The drawing under review shows one solid part. Ordinate dimensions are in mm from its lowest x, y, z. A direction names the side the tool comes from. Give positions to 0.01 mm unless a question says otherwise; leave off trailing zeros. Loops run counter-clockwise (first coordinate to the right, second up) from the corner with the lowest first, then second, coordinate; pieces in that order, holes last. Notation, with made-up numbers: M -6.75,33 L 44.25,33 A6 cw 44.25,41 Z; hole C -9.5,-2.5 d4. An arc over 180 degrees is marked long. Write item = value, one per line. Start each with the question number.
1. For the marked faces 4, 5 and 6, list the 3-axis set-ups (+Z, -Z, +X, -X, +Y, -Y) from which the entire face can be reached by the end or side of a thin tool; tool diameter is ignored.
2. We need section D-D on x = 9.5. Give the boundary of the cut face in (y, z).
3. We need section A-A on z = 8.5. Give the boundary of the cut face in (x, y), then the cut area to 3 significant figures.
4. For pin 1 (1.5 mm diameter, centred on x = 12, y = 42.5, fed in from -Z); pin 2 (12 mm diameter, centred on x = 11.5, y = 18.5, fed in from -Z); pin 3 (1 mm diameter, centred on x = 15, y = 39.5, fed in from +Z), all flat-tipped, find the tip position at first contact; note any pin that passes through.
5. Wall thickness on line 1 along X through (y, z) = (3.5, 8.5); line 2 along Z through (x, y) = (1.5, 19.5); line 3 along Z through (x, y) = (10.25, 11): over which ranges is each line inside the solid? List them lowest first. Write a range as from..to.
6. We need section C-C on y = 26. Give the boundary of the cut face in (x, z), then the cut area to 3 significant figures.
7. We need section B-B on x = 23.75. Give the boundary of the cut face in (y, z), then the cut area to 3 significant figures.
8. Draft analysis for pull direction Y (two halves, no side actions). For the marked faces 1, 2 and 3, state which applies: pulls with the +Y half, pulls with the -Y half, needs draft (parallel to the pull), parting line crosses it, or undercut.
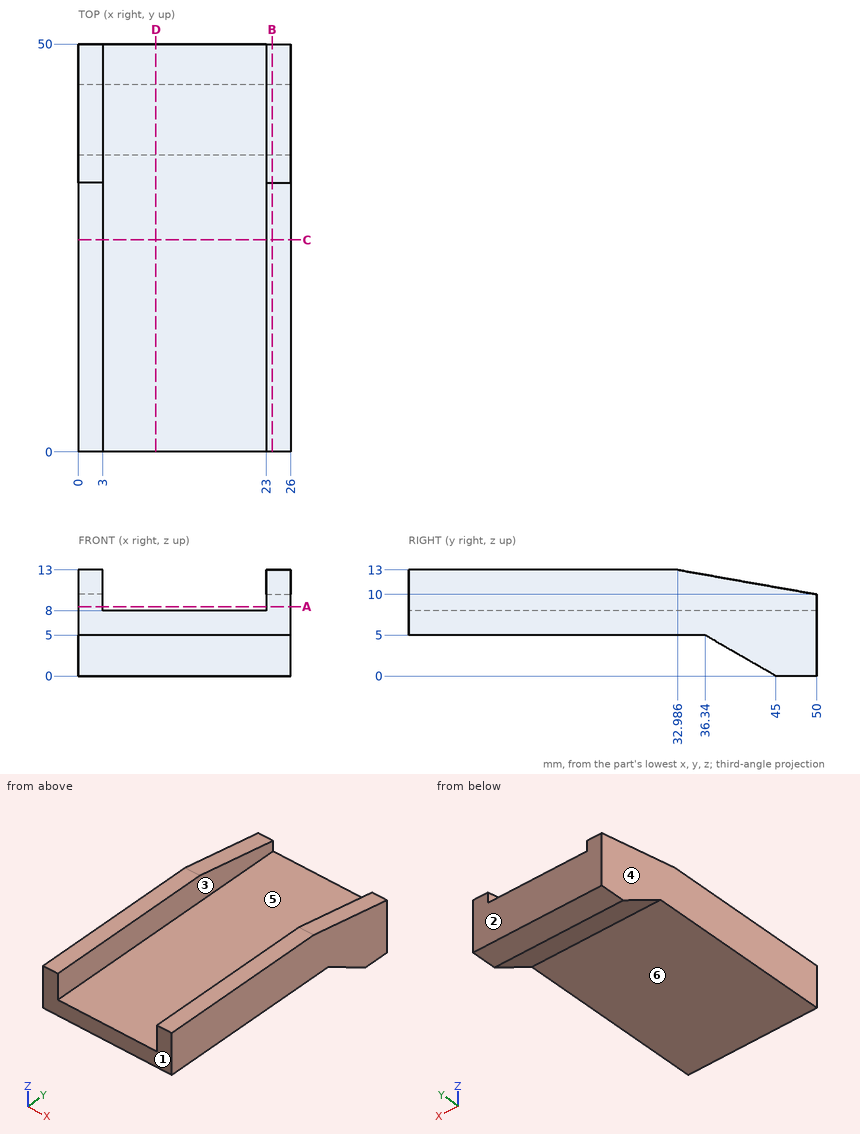
Final values:
q1.face_4 = +Z, -Z, -X, +Y, -Y
q1.face_5 = +Z, +Y, -Y
q1.face_6 = -Z, +X, -X, -Y
q2.outline = M 0,5 L 36.34,5 L 45,0 L 50,0 L 50,8 L 0,8 Z
q3.outline = M 0,0 L 3,0 L 3,50 L 0,50 Z; M 23,0 L 26,0 L 26,50 L 23,50 Z
q3.area = 300 mm²
q4.pin_1 = 1.01
q4.pin_2 = 5
q4.pin_3 = 8
q5.line_1 = 0..3, 23..26
q5.line_2 = 5..13
q5.line_3 = 5..8
q6.outline = M 0,5 L 26,5 L 26,13 L 23,13 L 23,8 L 3,8 L 3,13 L 0,13 Z
q6.area = 108 mm²
q7.outline = M 0,5 L 36.34,5 L 45,0 L 50,0 L 50,10 L 32.99,13 L 0,13 Z
q7.area = 421 mm²
q8.face_1 = pulls with the -Y half
q8.face_2 = pulls with the +Y half
q8.face_3 = needs draft
